Read the model definition and answer for the solid it produces. Units are mm, in the model's axes. A direction names the side the tool comes from. Coordinates: 2 decimals unless noted, no trailing zeros. Loops run counter-clockwise (first coordinate to the right, second up) from the corner with the lowest first, then second, coordinate; pieces in that order, holes last. Notation, with made-up numbers: (44, 84) -> (55, 84) arc R6 ccw to (55, 90) -> close; hole circle Ø3 at (3.5, -14). An arc over 180 degrees is marked (long way). Answer as a JSON object with one key per item and string values. Group by question number.
1) Consider probe 1 along Z at (x, y) = (0, 2.1); probe 2 along X at (y, z) = (2.75, -0.65); probe 3 along X at (y, z) = (1.75, 0.15). Determine where each line is inside the solid, lowest interval first. Write a range as [from, to].
2) Which of the six approach directions +Z, -Z, +X, -X, +Y, -Y give full straight-line access (tool end or side, diameter ignored) to faces 1 (the face through (1.29, 2.546, 2.024)), 2 (the face through (1.3, 2.3, 2.2)), 3 (the face through (-1.3, 2.3, 2.2))?
3) Flat-ended cylindrical pins translate along their axes: P1, Ø2, axis at x = 0, z = 0, coming from the -Y side; P2, Ø0.6, axis at x = -2.5, z = 0, coming from the +Y side. Find the tip coordinate at first contact, or state that the pin passes through.
4) Section A-A, the plane y = 1.2 is taken. Give the vertices of the cut face in (x, z).
from build123d import *

# Parameters (mm, degrees)
EXTRUDE_1_DEPTH     = 2.3
FILLET_1_R          = 0.1
SKETCH_2_R          = 2.4
EXTRUDE_2_DEPTH     = 3
FILLET_2_R          = 0.2
SKETCH_3_R          = 1.25
CUT_EXTRUDE_1_DEPTH = 12.8


with BuildPart() as part:
    # 草图1 → 凸台-拉伸1 (new body)
    with BuildSketch(Plane(origin=(0, 0, 0), x_dir=(1, 0, 0), z_dir=(0, 1, 0))):
        Polygon((1.443375673, -2.5), (2.886751346, 0), (1.443375673, 2.5), (-1.443375673, 2.5), (-2.886751346, 0), (-1.443375673, -2.5), align=None)
    extrude(amount=EXTRUDE_1_DEPTH)

    # 圆角1
    fillet_1_edges = [part.edges().sort_by_distance(p)[0] for p in [
        (2.165063509, 2.3, -1.25),
        (0, 2.3, -2.5),
        (-2.165063509, 2.3, -1.25),
        (-2.165063509, 2.3, 1.25),
        (0, 2.3, 2.5),
        (2.165063509, 2.3, 1.25),
    ]]
    fillet(fillet_1_edges, radius=FILLET_1_R)

    # 草图2 → 凸台-拉伸2 (add)
    with BuildSketch(Plane.XZ):
        Circle(SKETCH_2_R)
    extrude(amount=-EXTRUDE_2_DEPTH)

    # 圆角2
    fillet_2_edges = [part.edges().sort_by_distance(p)[0] for p in [
        (-2.4, 3, 0),
    ]]
    fillet(fillet_2_edges, radius=FILLET_2_R)

    # 草图3 → 切除-拉伸1 (cut)
    with BuildSketch(Plane.XZ):
        Circle(SKETCH_3_R)
    extrude(amount=-CUT_EXTRUDE_1_DEPTH, mode=Mode.SUBTRACT)


solid = part.part
Determined:
{
 "1": {"probe 1": "[-2.5, -1.25], [1.25, 2.5]", "probe 2": "[-2.31, -1.07], [1.07, 2.31]", "probe 3": "[-2.8, -1.24], [1.24, 2.8]"},
 "2": {"face 1": "+Y", "face 2": "+Z, +X, +Y", "face 3": "+Z, -X, +Y"},
 "3": {"P1": "through", "P2": "y = 3"},
 "4": {"outline": "(-2.89, 0) -> (-1.44, -2.5) -> (1.44, -2.5) -> (2.89, 0) -> (1.44, 2.5) -> (-1.44, 2.5) -> close; hole circle Ø2.5 at (0, 0)"}
}
